```python
from build123d import *

# Parameters (mm, degrees)
SKETCH2_W          = 50
SKETCH2_H          = 80
CUT_EXTRUDE1_DEPTH = 196.959179423
SKETCH3_W          = 70
SKETCH3_H          = 36
CUT_EXTRUDE2_DEPTH = 129.062484749
SKETCH5_W          = 30
SKETCH5_H          = 40
CUT_EXTRUDE3_DEPTH = 118.046999107


with BuildPart() as part:
    # Sketch1 → Revolve2 (revolve)
    with BuildSketch(Plane.XY):
        with BuildLine():
            Line((0, 0), (80, 0))
            ThreePointArc((80, 0), (56.568542495, 56.568542495), (0, 80))
            Line((0, 80), (0, 0))
        make_face()
    revolve(axis=Axis((0, 0, 0), (0, 1, 0)))

    # Sketch2 → Cut-Extrude1 (cut, through all)
    with BuildSketch(Plane.XY.offset(80)):
        with Locations((55, 40)):
            Rectangle(SKETCH2_W, SKETCH2_H)
        with Locations((-55, 40)):
            Rectangle(SKETCH2_W, SKETCH2_H)
    extrude(amount=-CUT_EXTRUDE1_DEPTH, mode=Mode.SUBTRACT)

    # Sketch3 → Cut-Extrude2 (cut, through all)
    with BuildSketch(Plane.ZY.offset(30)):
        with Locations((0, 18)):
            Rectangle(SKETCH3_W, SKETCH3_H)
    extrude(amount=-CUT_EXTRUDE2_DEPTH, mode=Mode.SUBTRACT)

    # Sketch5 → Cut-Extrude3 (cut, through all)
    with BuildSketch(Plane(origin=(0, 80, 0), x_dir=(-1, 0, 0), z_dir=(0, -1, 0))):
        with Locations((-0.075942229, -39.717020611)):
            Rectangle(SKETCH5_W, SKETCH5_H)
    extrude(amount=CUT_EXTRUDE3_DEPTH, mode=Mode.SUBTRACT)


solid = part.part
```
Work out the finished part from the listing and answer in its coordinate system (mm). A direction names the side the tool comes from. Give positions to 0.01 mm unless a question says otherwise; leave off trailing zeros. Order: outer loops, then holes, each group sorted by start corner. A loop starts at its lowest first (then second) coordinate and runs counter-clockwise, first axis right, second up. Notation, with made-up numbers: (-26, -12) - (19, -12) arc R15 ccw to (19, -4) - close; hole circle Ø2 at (3.25, 83). An arc over 180 degrees is marked (long way). One line per item, written item: value. Start each with the question number.
1. Which of the six approach directions +Z, -Z, +X, -X, +Y, -Y give full straight-line access (tool end or side, diameter ignored) to faces 1 (the face through (-14.924, 39, 40)), 2 (the face through (0, 0, -58)), 3 (the face through (22, 18, 35))?
2. For a pull along X with two mould halves and no side action, classify faces 4 (the face through (-30, 37, 1)), 5 (the face through (0, 57, 19.717)), 6 (the face through (0, 0, 62)) as released by +X, released by -X, zero draft, split by the parting line, or undercut.
3. Section C-C, the plane y = 46 is taken. Write down the section's boundary in (x, z).
4. Section A-A, the plane y = 13.5 is taken. Write down the section's boundary in (x, z).
5. Section B-B, the plane z = 45 is taken. Write down the section's boundary in (x, y), then the cut area to 3 significant figures.
6. Consider line 1 (X direction, y = 29, z = 59.5); line 2 (Z direction, x = 3, y = 18); line 3 (Z direction, x = -24, y = 9). Determine where each line is inside the solid, lowest interval first.
7. Section D-D, the plane x = -25.5 is taken. Write down the section's boundary in (y, z).
8. Each of these flat-tipped pins is pushed along its axis until it touches: pin 1 Ø5 at (x, z) = (19.5, -17) entering from +Y; pin 2 Ø2 at (x, z) = (10.5, 21) entering from +Y; pin 3 Ø16.5 at (x, y) = (19, 23) entering from -Z; pin 4 Ø8 at (x, z) = (15, 7.5) entering from -Y. Where does it stop, or does it pass through?
Filled sheet:
1. face 1: +Y, -Y
1. face 2: +Z, -Z, +X, -X, -Y
1. face 3: +X, -X, -Y
2. face 4: released by -X
2. face 5: undercut
2. face 6: zero draft
3. outline: (-30, -58.17) arc R65.45 ccw to (30, -58.17) - (30, 58.17) arc R65.45 ccw to (-30, 58.17) - close; hole (-14.92, 19.72) - (15.08, 19.72) - (15.08, 59.72) - (-14.92, 59.72) - close
4. outline: (-30, -72.92) arc R78.85 ccw to (30, -72.92) - (30, -35) - (-30, -35) - close; (-30, 35) - (-14.92, 35) - (-14.92, 59.72) - (15.08, 59.72) - (15.08, 35) - (30, 35) - (30, 72.92) arc R78.85 ccw to (-30, 72.92) - close
5. outline: (-30, 0) - (-14.92, 0) - (-14.92, 64.44) arc R66.14 ccw to (-30, 58.95) - close; (15.08, 0) - (30, 0) - (30, 58.95) arc R66.14 ccw to (15.08, 64.4) - close
5. area: 1,860 mm²
6. line 1: -30 to -14.92, 15.08 to 30
6. line 2: -77.89 to -35, 59.72 to 77.89
6. line 3: -75.78 to -35, 35 to 75.78
7. outline: (0, -75.83) arc R75.83 ccw to (0, 75.83) - (0, 35) - (36, 35) - (36, -35) - (0, -35) - close
8. pin 1: y = 76.51
8. pin 2: through
8. pin 3: z = -77.03
8. pin 4: y = 36
